Verification items for this drawing (mm, ordinates from the low corner). A direction names the side the tool comes from. Round coordinates to 2 decimals unless told otherwise and drop trailing zeros. Order: outer loops, then holes, each group sorted by start corner. A loop starts at its lowest first (then second) coordinate and runs counter-clockwise, first axis right, second up. Notation, with made-up numbers: M -15.75,23.25 L 15.25,23.25 A30 ccw 15.25,61.25 Z; hole C -8.5,64.5 d2. An arc over 180 degrees is marked long. Use CSV: the item, a comma, the result in double quotes. Start each with the question number.
Q1. Gauge pin test, flat end, axial feed: pin 1 Ø5 at (y, z) = (11, 11.5) entering from -X. Record the tip position at first contact, or that the pin passes through.
Q2. Sectioned sample at C-C (x = 41.5). Enter the section's corners in (y, z), and give its area (3 significant figures).
Q3. Sectioned sample at B-B (y = 25.5). Enter the section's corners in (x, z).
Q4. Set-up check for the marked faces 1, 2, 3, 4 and 5: record each of +Z, -Z, +X, -X, +Y, -Y from which the full face is reachable in a straight line by a thin tool's end or side.
Q5. Mould release check, pull along Y, two halves, no side actions. Record for the marked faces 6, 7, 8 and 9: +Y half, -Y half, draft (parallel to the pull), parting line (faces both ways), or undercut.
Q6. Sectioned sample at A-A (z = 3.75). Enter the section's corners in (x, y), and give its area (3 significant figures).
Q7. Sectioned sample at D-D (z = 6.75). Enter the section's corners in (x, y).
Q8. Scan lines: line 1 (X direction, y = 9, z = 8); line 2 (X direction, y = 31, z = 11.5); line 3 (Y direction, x = 23, z = 14.75). Record each from-to range of solid material in increasing order.
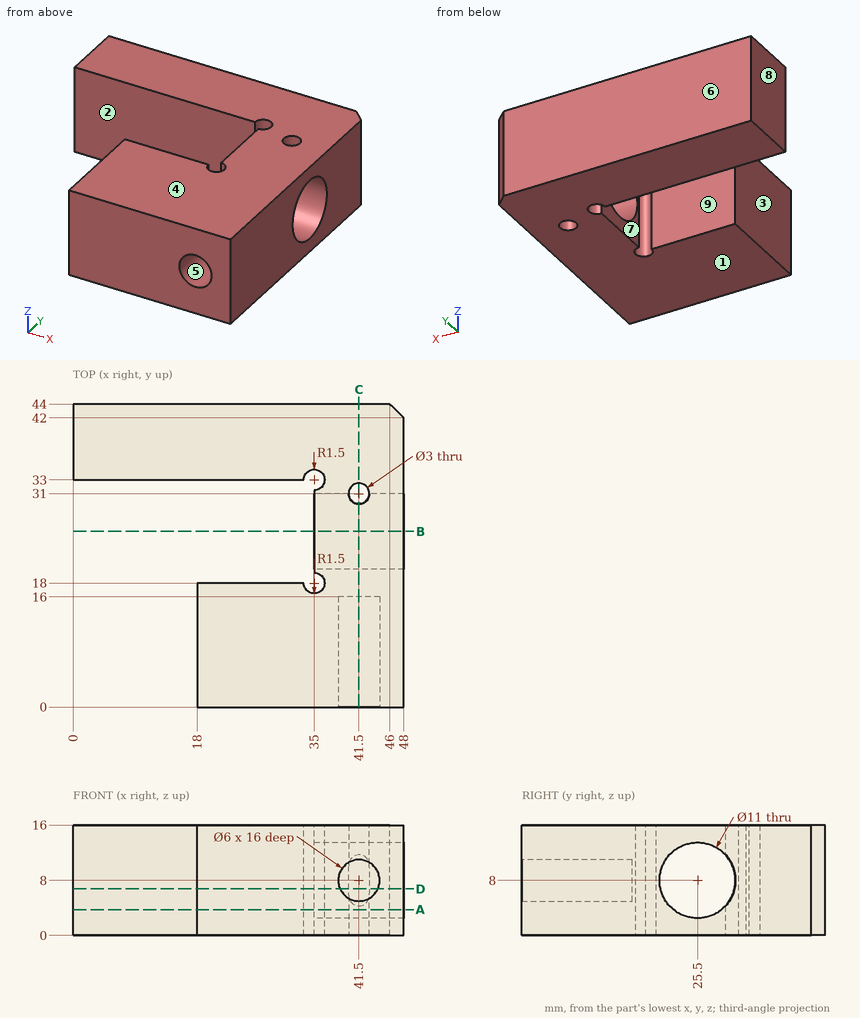
Verdict:
1,pin 1,"stops at x = 18"
2,outline,"M 0,0 L 29.5,0 L 29.5,4.23 A5.5 cw long 29.5,11.77 L 29.5,16 L 0,16 L 0,11 L 16,11 L 16,5 L 0,5 Z; M 32.5,0 L 44,0 L 44,16 L 32.5,16 Z"
2,area,"473 mm²"
3,outline,"M 35,0 L 48,0 L 48,2.5 L 35,2.5 Z; M 35,13.5 L 48,13.5 L 48,16 L 35,16 Z"
4,face 1,"-Z, +X, -X, +Y, -Y"
4,face 2,"+Z, -Z, -X"
4,face 3,"+Z, -Z, -X, -Y"
4,face 4,"+Z, +X, -X, +Y, -Y"
4,face 5,"-Y"
5,face 6,"+Y half"
5,face 7,"undercut"
5,face 8,"draft"
5,face 9,"undercut"
6,outline,"M 0,33 L 33.5,33 A1.5 cw long 35,31.5 L 35,28.99 L 48,28.99 L 48,42 L 46,44 L 0,44 Z; M 18,0 L 48,0 L 48,22.01 L 35,22.01 L 35,19.5 A1.5 cw long 33.5,18 L 18,18 Z; hole C 41.5,31 d3"
6,area,"1,150 mm²"
7,outline,"M 0,33 L 33.5,33 A1.5 cw long 35,31.5 L 35,30.86 L 40.01,30.86 A1.5 cw long 42.99,30.86 L 48,30.86 L 48,42 L 46,44 L 0,44 Z; M 18,0 L 38.77,0 L 38.77,16 L 44.23,16 L 44.23,0 L 48,0 L 48,20.14 L 35,20.14 L 35,19.5 A1.5 cw long 33.5,18 L 18,18 Z"
8,line 1,"x = 18 to 38.5, 44.5 to 48"
8,line 2,"x = 35 to 40, 43 to 48"
8,line 3,"y = 0 to 18, 33 to 44"
